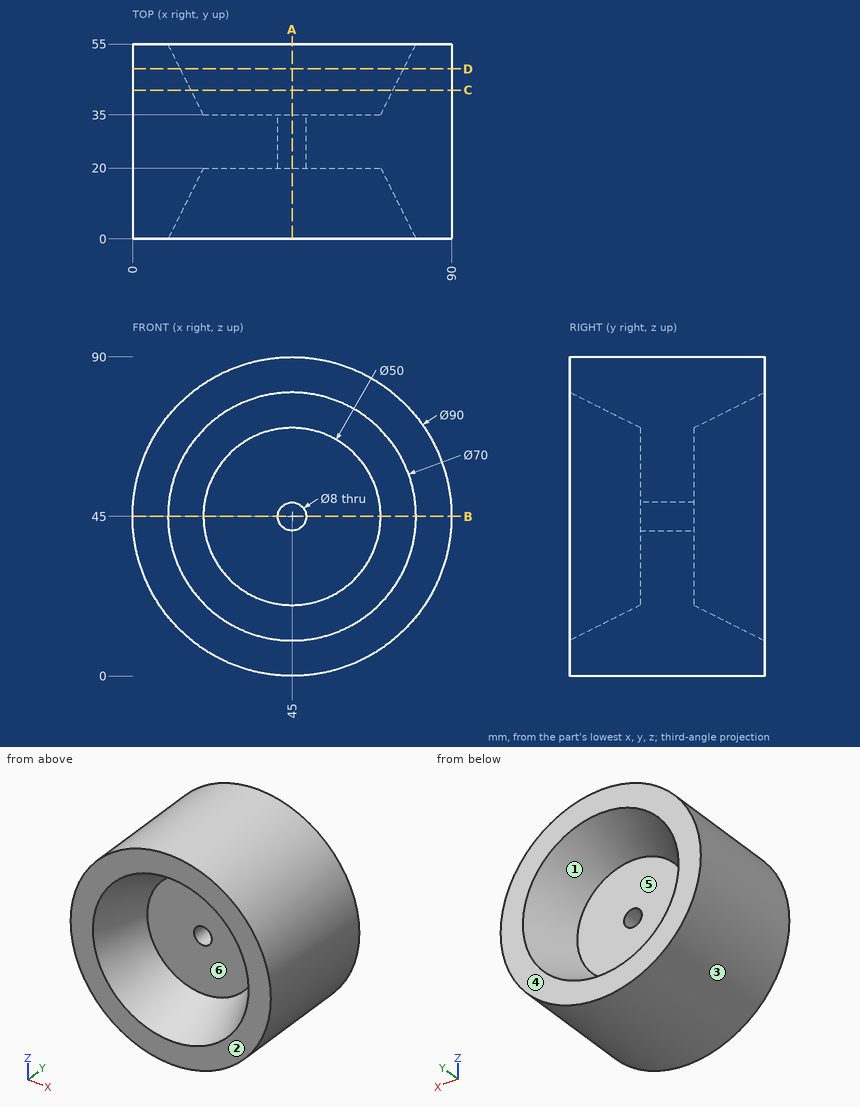
Job drawing, mm, ordinate dimensions from the low corner. One solid piece. A direction names the side the tool comes from. Give positions to 0.01 mm unless a question says otherwise; leave off trailing zeros. Write each loop counter-clockwise with the first axis right and the second up, starting at its lowest first coordinate (ties: lowest second). Pieces come first, ordered by that corner, then holes. Notation, with made-up numbers: (83, -6.5) - (112, -6.5) arc R20 ccw to (112, 3.5) - close; hole circle Ø11 at (-21, 82). An arc over 180 degrees is marked (long way). Use one line per item in the form item = value. Start each with the question number.
1. Drop flat-ended pins along their axis: pin 1 Ø10 at (x, z) = (72.5, 42.5) entering from +Y; pin 2 Ø1.5 at (x, y) = (44, 23.5) entering from -Z; pin 3 Ø2 at (x, y) = (54, 38) entering from +Z. Give the stop position or say it passes through.
2. Band-saw the part on D-D on y = 48. Write the cut outline in (x, z), plus the area to 3 significant figures.
3. Band-saw the part on A-A on x = 45. Write the cut outline in (y, z), plus the area to 3 significant figures.
4. Band-saw the part on B-B on z = 45. Write the cut outline in (x, y).
5. Two-plate mould, pull along X, no slides. Class the marked faces 1, 2 and 3: released by +X, released by -X, zero draft, split by the parting line, or undercut.
6. 3-axis set-ups, long thin cutter, end or side, ignore diameter. For the marked faces 4, 5 and 6: which of +Z, -Z, +X, -X, +Y, -Y reach the whole face in a straight line?
7. Probe line 1 (X direction, y = 30, z = 45); line 2 (Y direction, x = 36, z = 33.5); line 3 (X direction, y = 14, z = 37.5). List the from-to ranges inside material, lowest first. Write a range as [from, to].
8. Band-saw the part on C-C on y = 42. Write the cut outline in (x, z), plus the area to 3 significant figures.
Conclusion:
q1.pin_1 = 50.23
q1.pin_2 = 0
q1.pin_3 = 89.28
q2.outline = circle Ø90 at (45, 45); hole circle Ø63 at (45, 45)
q2.area = 3,240 mm²
q3.outline = (0, 0) - (55, 0) - (55, 10) - (35, 20) - (35, 41) - (20, 41) - (20, 20) - (0, 10) - close; (0, 80) - (20, 70) - (20, 49) - (35, 49) - (35, 70) - (55, 80) - (55, 90) - (0, 90) - close
q3.area = 2,430 mm²
q4.outline = (0, 0) - (10, 0) - (20, 20) - (41, 20) - (41, 35) - (20, 35) - (10, 55) - (0, 55) - close; (49, 20) - (70, 20) - (80, 0) - (90, 0) - (90, 55) - (80, 55) - (70, 35) - (49, 35) - close
q5.face_1 = undercut
q5.face_2 = zero draft
q5.face_3 = split by the parting line
q6.face_4 = +Z, -Z, +X, -X, +Y
q6.face_5 = +Y
q6.face_6 = -Y
q7.line_1 = [0, 41], [49, 90]
q7.line_2 = [20, 35]
q7.line_3 = [0.63, 18.02], [71.98, 89.37]
q8.outline = circle Ø90 at (45, 45); hole circle Ø57 at (45, 45)
q8.area = 3,810 mm²
